For this review, take the finished solid that the model builds, in its own axes (mm). Give positions to 0.01 mm unless a question says otherwise; leave off trailing zeros. Order: outer loops, then holes, each group sorted by start corner. A loop starts at its lowest first (then second) coordinate and runs counter-clockwise, first axis right, second up. Notation, with made-up numbers: M 65.25,76.25 L 123.25,76.25 A25 cw 123.25,100.25 Z; hole C 13,22 d8. An arc over 180 degrees is marked long. Use CSV: the item, a comma, the result in double quotes. Start each with the question number.
(1) Consider section B-B (z = 0). Write out the cut boundary in (x, y), and give its area (4 significant figures).
(2) Wall thickness on L1, parallel to X at y = 342.5, z = -5; L2, parallel to X at y = -406, z = 8; L3, parallel to Z at x = 11.7, y = 517: over which ranges is each line inside the solid? List them lowest first. Write a range as from..to.
(3) Consider section C-C (x = -1.75). Write out the cut boundary in (y, z).
(4) Consider section A-A (y = 204.5). Write out the cut boundary in (x, z), and give its area (3 significant figures).
(5) Clearance check with a flat-ended pin moving along its axis: P1, Ø14.5, axis at y = -517, z = 0, coming from the -X side. State where the tip first meets the part, or that it passes through.
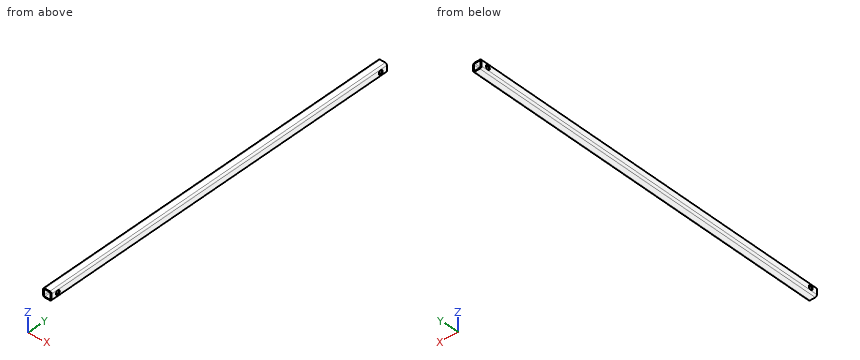
```python
from build123d import *

# Parameters (mm, degrees)
F1_DEPTH = 537
F2_R     = 6.25
F3_DEPTH = 25.001


with BuildPart() as f1:
    # F0 (on Front) → F1 (new body, symmetric)
    with BuildSketch(Plane.XZ):
        with BuildLine():
            ThreePointArc((12.5, 7.5), (11.035534, 11.035534), (7.5, 12.5))
            Line((7.5, 12.5), (-7.5, 12.5))
            ThreePointArc((-7.5, 12.5), (-11.035534, 11.035534), (-12.5, 7.5))
            Line((-12.5, 7.5), (-12.5, -7.5))
            ThreePointArc((-12.5, -7.5), (-11.035534, -11.035534), (-7.5, -12.5))
            Line((-7.5, -12.5), (7.5, -12.5))
            ThreePointArc((7.5, -12.5), (11.035534, -11.035534), (12.5, -7.5))
            Line((12.5, -7.5), (12.5, 7.5))
        make_face()
        with BuildLine():
            Line((-7.5, 10), (7.5, 10))
            ThreePointArc((7.5, 10), (9.267767, 9.267767), (10, 7.5))
            Line((10, 7.5), (10, -7.5))
            ThreePointArc((10, -7.5), (9.267767, -9.267767), (7.5, -10))
            Line((7.5, -10), (-7.5, -10))
            ThreePointArc((-7.5, -10), (-9.267767, -9.267767), (-10, -7.5))
            Line((-10, -7.5), (-10, 7.5))
            ThreePointArc((-10, 7.5), (-9.267767, 9.267767), (-7.5, 10))
        make_face(mode=Mode.SUBTRACT)
    extrude(amount=F1_DEPTH, both=True)

    # F2 (on face) → F3 (cut, through all)
    with BuildSketch(Plane.YZ.offset(12.5)):
        with Locations((-517, 0)):
            Circle(F2_R)
        with Locations((517, 0)):
            Circle(F2_R)
    extrude(amount=-F3_DEPTH, mode=Mode.SUBTRACT)


solid = f1.part
```
Check result:
1,outline,"M -12.5,-537 L -10,-537 L -10,-523.25 L -12.5,-523.25 Z; M -12.5,-510.75 L -10,-510.75 L -10,510.75 L -12.5,510.75 Z; M -12.5,523.25 L -10,523.25 L -10,537 L -12.5,537 Z; M 10,-537 L 12.5,-537 L 12.5,-523.25 L 10,-523.25 Z; M 10,-510.75 L 12.5,-510.75 L 12.5,510.75 L 10,510.75 Z; M 10,523.25 L 12.5,523.25 L 12.5,537 L 10,537 Z"
1,area,"5,245 mm^2"
2,L1,"x = -12.5..-10, 10..12.5"
2,L2,"x = -12.47..-9.95, 9.95..12.47"
2,L3,"z = -10.21..-6.25, 6.25..10.21"
3,outline,"M -537,-12.5 L 537,-12.5 L 537,-10 L -537,-10 Z; M -537,10 L 537,10 L 537,12.5 L -537,12.5 Z"
4,outline,"M -12.5,-7.5 A5 ccw -7.5,-12.5 L 7.5,-12.5 A5 ccw 12.5,-7.5 L 12.5,7.5 A5 ccw 7.5,12.5 L -7.5,12.5 A5 ccw -12.5,7.5 Z; hole M -10,-7.5 A2.5 ccw -7.5,-10 L 7.5,-10 A2.5 ccw 10,-7.5 L 10,7.5 A2.5 ccw 7.5,10 L -7.5,10 A2.5 ccw -10,7.5 Z"
4,area,"209 mm^2"
5,P1,"stops at x = -12.5"
